The listing builds one solid part. Answer for the finished solid, in the listing's coordinates (mm). Give positions to 0.01 mm unless a question says otherwise; leave off trailing zeros. Write each loop counter-clockwise with the first axis right and the second up, starting at its lowest first coordinate (ties: lowest second). Pieces come first, ordered by that corner, then holes. Notation, with made-up numbers: (5, 75.25) -> (42, 75.25) arc R23 cw to (42, 92.25) -> close; hole circle Ø11 at (-19, 5). An arc over 180 degrees is marked (long way). Put each result on its own line as item: value. Start each with the question number.
1) A cutting plane is placed at B-B (x = -9.5). Write down the section's boundary in (y, z).
2) A flat-ended cylindrical pin translates along its axis: pin 1 Ø5 at (x, y) = (14.3, 17.7) entering from +Z. Find the tip coordinate at first contact, or state that the pin passes through.
3) A cutting plane is placed at A-A (z = 1.45). Write down the section's boundary in (x, y), then the cut area to 3 significant figures.
4) Find the intervals of material crossed by line 1 along Y through (x, z) = (0, 1.4); line 2 along X through (y, z) = (4, 2.85); line 3 along Y through (x, z) = (-13, 2.8), in increasing order. Write a range as from..to.
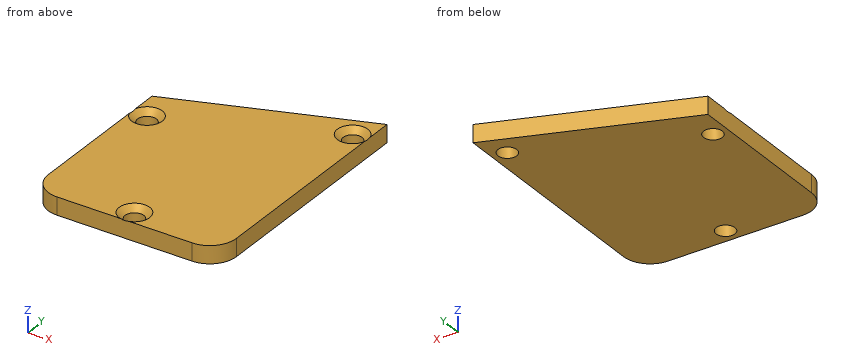
from build123d import *

# Parameters (mm, degrees)
DODANIE_WYCI_GNI_CIE1_DEPTH = 3
SZKIC2_R                    = 1.6
WYTNIJ_WYCI_GNI_CIE1_DEPTH  = 3
SFAZOWANIE1_SIZE            = 1


with BuildPart() as part:
    # Szkic1 → Dodanie-wyciągnięcie1 (new body)
    with BuildSketch(Plane.XY):
        with BuildLine():
            Line((16.79955852, 22.699230769), (-15.20044148, 10.769230769))
            Line((-15.20044148, 10.769230769), (-15.20044148, -15.560769231))
            ThreePointArc((-15.20044148, -15.560769231), (-13.882421995, -18.742749746), (-10.70044148, -20.060769231))
            Line((-10.70044148, -20.060769231), (12.29955852, -20.060769231))
            ThreePointArc((12.29955852, -20.060769231), (15.481539035, -18.742749746), (16.79955852, -15.560769231))
            Line((16.79955852, -15.560769231), (16.79955852, 22.699230769))
        make_face()
    extrude(amount=DODANIE_WYCI_GNI_CIE1_DEPTH)

    # Szkic2 → Wytnij-wyciągnięcie1 (cut)
    with BuildSketch(Plane.XY.offset(3)):
        with Locations((-12.70044148, 5.769230769)):
            Circle(SZKIC2_R)
        with Locations((14.29955852, 17.699230769)):
            Circle(SZKIC2_R)
        with Locations((0.79955852, -17.560769231)):
            Circle(SZKIC2_R)
    extrude(amount=-WYTNIJ_WYCI_GNI_CIE1_DEPTH, mode=Mode.SUBTRACT)

    # Sfazowanie1
    # the kernel refuses this chamfer: 1 mm, written as the material it takes off along each edge
    with BuildSketch(Plane(origin=(-12.70044148, 5.769230769, 3), x_dir=(1, 0, 0), z_dir=(0, -1, 0))) as sfazowanie1_piece_1:
        Polygon((1.6 + SFAZOWANIE1_SIZE, 0), (1.6, -SFAZOWANIE1_SIZE), (1.6, 0), align=None)
    revolve(axis=Axis((-12.70044148, 5.769230769, 3), (0, 0, 1)), mode=Mode.SUBTRACT)
    with BuildSketch(Plane(origin=(14.29955852, 17.699230769, 3), x_dir=(1, 0, 0), z_dir=(0, -1, 0))) as sfazowanie1_piece_2:
        Polygon((1.6 + SFAZOWANIE1_SIZE, 0), (1.6, -SFAZOWANIE1_SIZE), (1.6, 0), align=None)
    revolve(axis=Axis((14.29955852, 17.699230769, 3), (0, 0, 1)), mode=Mode.SUBTRACT)
    with BuildSketch(Plane(origin=(0.79955852, -17.560769231, 3), x_dir=(1, 0, 0), z_dir=(0, -1, 0))) as sfazowanie1_piece_3:
        Polygon((1.6 + SFAZOWANIE1_SIZE, 0), (1.6, -SFAZOWANIE1_SIZE), (1.6, 0), align=None)
    revolve(axis=Axis((0.79955852, -17.560769231, 3), (0, 0, 1)), mode=Mode.SUBTRACT)


solid = part.part
Reply:
1. outline: (-20.06, 0) -> (12.89, 0) -> (12.89, 3) -> (-20.06, 3) -> close
2. pin 1: stops at z = 2.9
3. outline: (-15.2, -15.56) arc R4.5 ccw to (-10.7, -20.06) -> (12.3, -20.06) arc R4.5 ccw to (16.8, -15.56) -> (16.8, 22.7) -> (-15.2, 10.77) -> close; hole circle Ø3.2 at (-12.7, 5.77); hole circle Ø3.2 at (0.8, -17.56); hole circle Ø3.2 at (14.3, 17.7)
3. area: 1,140 mm2
4. line 1: y = -20.06..-18.95, -16.17..16.44
4. line 2: x = -15.2..-14.4, -11.01..16.8
4. line 3: y = -19.43..3.39, 8.15..11.59
